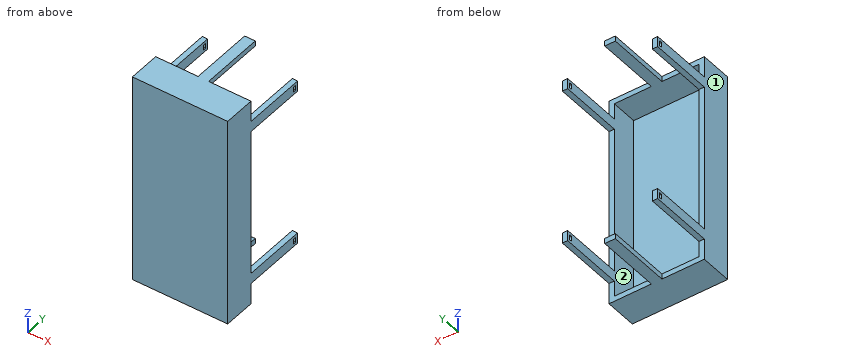
Autodesk Inventor part; units mm, degrees
ref_plane "YZ Plane" through (0, 0, 0) normal (1, 0, 0) x (0, 1, 0)
ref_plane "XZ Plane" through (0, 0, 0) normal (0, 1, 0) x (-1, 0, 0)
ref_plane "XY Plane" through (0, 0, 0) normal (0, 0, 1) x (1, 0, 0)
sketch "Sketch1" plane through (0, 0, 0) normal (0, 1, 0) x (-1, 0, 0)
  line L0 (0, 0) -> (3.175, 0)
  line L1 (3.175, 0) -> (3.175, -3.175)
  line L2 (3.175, -3.175) -> (0, -3.175)
  line L3 (0, -3.175) -> (0, 0)
  line L4 (0, 0) -> (6.35, 0)
  line L5 (0, -6.35) -> (0, 0)
  line L6 (3.175, 0) -> (50.8, 0)
  line L7 (50.8, 0) -> (50.8, -3.175)
  line L8 (50.8, -3.175) -> (3.175, -3.175)
  line L9 (3.175, -3.175) -> (3.175, 0)
  line L10 (50.8, 0) -> (57.15, 0)
  line L11 (57.15, 0) -> (57.15, -6.35)
  line L12 (57.15, 0) -> (53.975, 0)
  line L13 (53.975, 0) -> (53.975, -3.175)
  line L14 (53.975, -3.175) -> (57.15, -3.175)
  line L15 (57.15, -3.175) -> (57.15, 0)
  line L16 (53.975, -120.65) -> (53.975, -123.825)
  line L17 (53.975, -123.825) -> (50.8, -123.825)
  line L18 (57.15, -120.65) -> (57.15, -127)
  line L19 (57.15, -127) -> (50.8, -127)
  line L20 (3.175, -120.65) -> (3.175, -123.825)
  line L21 (3.175, -123.825) -> (6.35, -123.825)
  line L22 (0, -120.65) -> (0, -127)
  line L23 (0, -127) -> (6.35, -127)
  line L24 (53.975, -127) -> (57.15, -127)
  line L25 (57.15, -127) -> (57.15, 0)
  line L26 (57.15, 0) -> (53.975, 0)
  line L27 (53.975, 0) -> (53.975, -127)
  line L28 (50.8, -3.175) -> (57.15, -3.175)
  line L29 (57.15, -3.175) -> (57.15, 0)
  line L30 (57.15, 0) -> (50.8, 0)
  line L31 (50.8, 0) -> (50.8, -3.175)
  line L32 (50.8, -127) -> (6.35, -127)
  line L33 (6.35, -127) -> (6.35, -123.825)
  line L34 (6.35, -123.825) -> (50.8, -123.825)
  line L35 (50.8, -123.825) -> (50.8, -127)
  line L36 (0, -120.65) -> (3.175, -120.65)
  line L37 (3.175, -120.65) -> (3.175, -6.35)
  line L38 (3.175, -6.35) -> (0, -6.35)
  line L39 (0, -6.35) -> (0, -120.65)
  line L40 (3.175, -6.35) -> (3.175, -3.175)
  line L41 (3.175, -3.175) -> (6.35, -3.175)
  line L42 (53.975, -123.825) -> (57.15, -123.825)
  line L43 (57.15, -123.825) -> (57.15, -120.65)
  line L44 (57.15, -120.65) -> (53.975, -120.65)
  line L45 (53.975, -120.65) -> (53.975, -123.825)
  line L46 (0, -127) -> (3.175, -127)
  line L47 (3.175, -127) -> (3.175, -123.825)
  line L48 (3.175, -123.825) -> (0, -123.825)
  line L49 (0, -123.825) -> (0, -127)
  line L50 (3.175, -3.175) -> (6.35, -3.175)
  line L51 (6.35, -3.175) -> (6.35, 0)
  line L52 (6.35, 0) -> (3.175, 0)
  line L53 (3.175, 0) -> (3.175, -3.175)
  line L54 (57.15, -3.175) -> (53.975, -3.175)
  line L55 (53.975, -3.175) -> (53.975, -6.35)
  line L56 (53.975, -6.35) -> (57.15, -6.35)
  line L57 (57.15, -6.35) -> (57.15, -3.175)
  line L58 (57.15, -6.35) -> (53.975, -6.35)
  line L59 (53.975, -6.35) -> (53.975, -120.65)
  line L60 (53.975, -120.65) -> (57.15, -120.65)
  line L61 (57.15, -120.65) -> (57.15, -6.35)
  line L62 (3.175, -3.175) -> (0, -3.175)
  line L63 (0, -3.175) -> (0, -6.35)
  line L64 (0, -6.35) -> (3.175, -6.35)
  line L65 (3.175, -6.35) -> (3.175, -3.175)
  line L66 (3.175, -123.825) -> (0, -123.825)
  line L67 (0, -123.825) -> (0, -120.65)
  line L68 (0, -120.65) -> (3.175, -120.65)
  line L69 (3.175, -120.65) -> (3.175, -123.825)
  line L70 (3.175, -123.825) -> (6.35, -123.825)
  line L71 (6.35, -123.825) -> (6.35, -127)
  line L72 (6.35, -127) -> (3.175, -127)
  line L73 (3.175, -127) -> (3.175, -123.825)
  line L74 (53.975, -123.825) -> (50.8, -123.825)
  line L75 (50.8, -123.825) -> (50.8, -127)
  line L76 (50.8, -127) -> (53.975, -127)
  line L77 (53.975, -127) -> (53.975, -123.825)
  line L78 (57.15, -120.65) -> (53.975, -120.65)
  line L79 (53.975, -120.65) -> (53.975, -123.825)
  line L80 (53.975, -123.825) -> (57.15, -123.825)
  line L81 (57.15, -123.825) -> (57.15, -120.65)
  dimension "d2" = 3.175
  dimension "d3" = 3.175
  dimension "d7" = 6.35
  dimension "d8" = 3.175
  dimension "d9" = 3.175
  dimension "d10" = 3.175
  dimension "d11" = 3.175
  dimension "d12" = 6.35
  dimension "d13" = 6.35
  dimension "d14" = 3.175
  dimension "d15" = 3.175
  dimension "d16" = 6.35
  dimension "d17" = 6.35
  dimension "d18" = 3.175
extrude "Extrusion1" add sketch "Sketch1" along normal blind 19.05 contours L0 L1 L2 L3 | L4 L51 L8 L1 | L2 L40 L38 L5 | L6 L7 L8 L51 | L38 L37 L36 L39 | L10 L13 L28 L7 | L36 L20 L48 L22 | L10 L11 L14 L13 | L48 L47 L23 L22 | L14 L11 L56 L27 | L21 L33 L23 L47 | L56 L25 L44 L27 | L34 L35 L32 L33 | L44 L18 L42 L16 | L17 L27 L19 L35 | L42 L18 L19 L27
sketch "Sketch2" plane through (0, 0, 0) normal (0, -1, 0) x (1, 0, 0)
  line L0 (-3.175, -3.175) -> (-53.975, -3.175)
  line L1 (-53.975, -123.825) -> (-3.175, -123.825)
  line L2 (-3.175, -123.825) -> (-3.175, -3.175)
  line L3 (-3.175, -3.175) -> (-53.975, -3.175)
  line L4 (-53.975, -3.175) -> (-53.975, -123.825)
  point P0 (0, 0)
extrude "Extrusion2" add sketch "Sketch2" against normal blind 3.175
sketch "Sketch3" plane through (0, 19.05, 0) normal (0, 1, 0) x (1, 0, 0)
  line L0 (0, 127) -> (-57.15, 127)
  line L1 (-57.15, 0) -> (0, 0)
  line L2 (-3.175, 123.825) -> (-53.975, 123.825)
  line L3 (-57.15, 127) -> (-57.15, 0)
  line L4 (-3.175, 3.175) -> (-53.975, 3.175)
  line L5 (-3.175, 123.825) -> (-3.175, 3.175)
  line L6 (-53.975, 3.175) -> (-53.975, 123.825)
  line L7 (0, 0) -> (0, 127)
  line L8 (0, 114.3) -> (-3.175, 114.3)
  line L9 (-3.175, 114.3) -> (0, 114.3)
  line L10 (0, 114.3) -> (0, 107.95)
  line L11 (0, 107.95) -> (-3.175, 107.95)
  line L12 (-3.175, 107.95) -> (-3.175, 114.3)
  line L13 (0, 0) -> (0, 12.7)
  line L14 (0, 12.7) -> (-3.175, 12.7)
  line L15 (-3.175, 12.7) -> (0, 12.7)
  line L16 (0, 12.7) -> (0, 19.05)
  line L17 (0, 19.05) -> (-3.175, 19.05)
  line L18 (-3.175, 19.05) -> (-3.175, 12.7)
  line L19 (-53.975, 12.7) -> (-57.15, 12.7)
  line L20 (-57.15, 12.7) -> (-57.15, 19.05)
  line L21 (-57.15, 19.05) -> (-53.975, 19.05)
  line L22 (-53.975, 19.05) -> (-53.975, 12.7)
  line L23 (-53.975, 114.3) -> (-57.15, 114.3)
  line L24 (-57.15, 114.3) -> (-57.15, 107.95)
  line L25 (-57.15, 107.95) -> (-53.975, 107.95)
  line L26 (-53.975, 107.95) -> (-53.975, 114.3)
  line L27 (-31.75, 123.825) -> (-25.4, 123.825)
  line L28 (-25.4, 123.825) -> (-25.4, 127)
  line L29 (-25.4, 127) -> (-31.75, 127)
  line L30 (-31.75, 127) -> (-31.75, 123.825)
  line L31 (-31.75, 123.825) -> (-25.4, 127) construction
  line L32 (-25.4, 123.825) -> (-31.75, 127) construction
  line L33 (-31.75, 3.175) -> (-25.4, 3.175)
  line L34 (-25.4, 3.175) -> (-25.4, 0)
  line L35 (-25.4, 0) -> (-31.75, 0)
  line L36 (-31.75, 0) -> (-31.75, 3.175)
  line L37 (-31.75, 3.175) -> (-25.4, 0) construction
  line L38 (-25.4, 3.175) -> (-31.75, 0) construction
  point P0 (-28.575, 125.4125)
  point P1 (-28.575, 1.5875)
  dimension "d23" = 127
  dimension "d24" = 57.15
  dimension "d45" = 6.35
  dimension "d46" = 3.175
  dimension "d49" = 3.175
  dimension "d50" = 6.35
  dimension "d51" = 6.35
  dimension "d52" = 6.35
  dimension "d53" = 6.35
  dimension "d54" = 3.175
  dimension "d55" = 0
  dimension "d56" = 28.575
  dimension "d57" = 6.35
  dimension "d58" = 3.175
  dimension "d59" = 0
  dimension "d60" = 28.575
  dimension "d71" = 12.7
  dimension "d72" = 12.7
  dimension "d73" = 12.7
  dimension "d74" = 12.7
extrude "Extrusion3" add sketch "Sketch3" along normal blind 38.1 contours L28 L2 L30 L0 | L7 L11 L5 L8 | L7 L14 L5 L17 | L23 L6 L25 L3 | L21 L6 L19 L3 | L1 L36 L4 L34
sketch "Sketch5" plane through (0, 0, 0) normal (1, 0, 0) x (0, 0, -1)
  line L0 (114.3, 19.05) -> (114.3, 57.15)
  line L1 (107.95, 19.05) -> (107.95, 57.15)
  line L2 (109.5375, 55.5625) -> (112.7125, 55.5625)
  line L3 (112.7125, 55.5625) -> (112.7125, 53.975)
  line L4 (112.7125, 53.975) -> (109.5375, 53.975)
  line L5 (109.5375, 53.975) -> (109.5375, 55.5625)
  line L6 (107.95, 57.15) -> (114.3, 57.15)
  line L7 (14.2875, 53.975) -> (17.4625, 53.975)
  line L8 (17.4625, 53.975) -> (17.4625, 55.5625)
  line L9 (17.4625, 55.5625) -> (14.2875, 55.5625)
  line L10 (14.2875, 55.5625) -> (14.2875, 53.975)
  line L11 (12.7, 19.05) -> (12.7, 57.15)
  line L12 (12.7, 57.15) -> (19.05, 57.15)
  point P0 (0, 0)
  dimension "d61" = 6.35
  dimension "d62" = 3.175
  dimension "d63" = 1.5875
  dimension "d64" = 1.5875
  dimension "d66" = 1.5875
  dimension "d67" = 3.175
  dimension "d68" = 1.5875
  dimension "d88" = 1.5875
  dimension "d89" = 1.5875
extrude "Extrusion4" cut sketch "Sketch5" against normal blind 25374.6
CAD build for the part. Positions are in the model's coordinates, mm. Face numbers are marked on the shaded views. A direction names the side the tool comes from. Give positions to 0.01 mm unless a question says otherwise; leave off trailing zeros. Order: outer loops, then holes, each group sorted by start corner. A loop starts at its lowest first (then second) coordinate and runs counter-clockwise, first axis right, second up.
(1) Tool access for the marked faces 1 and 2: list every direction of +Z, -Z, +X, -X, +Y, -Y with a clear straight run to the whole face (end or side of a thin tool).
(2) Saw through at B-B, the plane z = -39. Give the cut face in (x, y) (3 decimals).
(3) Saw through at A-A, the plane y = 46.5. Give the cut face in (x, z) (3 decimals).
(4) Saw through at C-C, the plane x = -27.5. Give the cut face in (y, z) (3 decimals).
(5) Saw through at D-D, the plane y = 12.5. Give the cut face in (x, z) (3 decimals), then the cut area to 3 significant figures.
(6) Drill centre lines: L1, parallel to X at y = 7, z = -77 (3 decimals); L2, parallel to Z at x = -42, y = 18 (3 decimals); L3, parallel to Z at x = -3, y = 34. Where is each one in solid material? Low to high.
(7) Flat gauge pins, fed straight in: pin 1 (1.6 mm diameter, centred on y = 36.5, z = -1, fed in from +X); pin 2 (2.5 mm diameter, centred on x = -56, y = 33.5, fed in from -Z); pin 3 (1.3 mm diameter, centred on x = -56, y = 55, fed in from +Z). Where does each tip first touch, or does it go through?
Results found:
1. face 1: +Z, -Z, -X, +Y, -Y
1. face 2: +Y
2. outline: (-57.15, 0) - (0, 0) - (0, 19.05) - (-3.175, 19.05) - (-3.175, 3.175) - (-53.975, 3.175) - (-53.975, 19.05) - (-57.15, 19.05) - close
3. outline: (-57.15, -114.3) - (-53.975, -114.3) - (-53.975, -107.95) - (-57.15, -107.95) - close; (-57.15, -19.05) - (-53.975, -19.05) - (-53.975, -12.7) - (-57.15, -12.7) - close; (-31.75, -127) - (-25.4, -127) - (-25.4, -123.825) - (-31.75, -123.825) - close; (-31.75, -3.175) - (-25.4, -3.175) - (-25.4, 0) - (-31.75, 0) - close; (-3.175, -114.3) - (0, -114.3) - (0, -107.95) - (-3.175, -107.95) - close; (-3.175, -19.05) - (0, -19.05) - (0, -12.7) - (-3.175, -12.7) - close
4. outline: (0, -127) - (57.15, -127) - (57.15, -123.825) - (3.175, -123.825) - (3.175, -3.175) - (57.15, -3.175) - (57.15, 0) - (0, 0) - close
5. outline: (-57.15, -127) - (0, -127) - (0, 0) - (-57.15, 0) - close; hole (-53.975, -123.825) - (-3.175, -123.825) - (-3.175, -3.175) - (-53.975, -3.175) - close
5. area: 1,130 mm2
6. L1: x = -57.15 to -53.975, -3.175 to 0
6. L2: z = -127 to -123.825, -3.175 to 0
6. L3: z = -114.3 to -107.95, -19.05 to -12.7
7. pin 1: stops at x = -25.4
7. pin 2: stops at z = -114.3
7. pin 3: stops at z = -12.7
